from build123d import *

# Parameters (mm, degrees)
F0_R     = 4.5
F0_R_2   = 3
F1_DEPTH = 1.9
F0_R_3   = 6.5
F0_R_4   = 2
F2_DEPTH = 2
F3_R     = 1.75
F5_SIZE  = 0.09999


# Not quite as in the source:
# - a fillet or chamfer is up to 0.001 mm smaller than in the source, because OpenCascade refuses the exact size


with BuildPart() as f1:
    # F0 (on Front) → F1 (new body, symmetric)
    with BuildSketch(Plane.XZ):
        Circle(F0_R)
        Circle(F0_R_2, mode=Mode.SUBTRACT)
    extrude(amount=F1_DEPTH, both=True)

    # F0 (on Front) → F2 (join, symmetric)
    with BuildSketch(Plane.XZ):
        Circle(F0_R_3)
        Circle(F0_R, mode=Mode.SUBTRACT)
        Circle(F0_R_2)
        Circle(F0_R_4, mode=Mode.SUBTRACT)
    extrude(amount=F2_DEPTH, both=True)

    # F4: sweep along a path in F4_path
    with BuildLine(Plane(origin=(6.5, -2, 0), x_dir=(0, 0, -1), z_dir=(0, 1, 0))) as f4_path:
        CenterArc((0, 6.5), 6.5, 0, 360)
    # F3 (on Right) → F4 (sweep, cut)
    with BuildSketch(Plane.YZ):
        with Locations((0, 7.25)):
            Circle(F3_R)
    sweep(path=f4_path.line, mode=Mode.SUBTRACT)

    # F5 (size 0.1 in the source; OpenCascade refuses exactly that, so slightly less here)
    f5_edges = [f1.edges().sort_by_distance(p)[0] for p in [
        (-6.5, -2, 0),
        (-4.5, -2, 0),
        (-3, -1.9, 0),
        (-2, -2, 0),
        (-2, 2, 0),
        (-3, 2, 0),
        (-4.5, 2, 0),
        (-6.5, 2, 0),
    ]]
    chamfer(f5_edges, length=F5_SIZE)


solid = f1.part
Can you work these out from the model? Positions are in its coordinate system, mm. A direction names the side the tool comes from. Give positions to 0.01 mm unless a question says otherwise; leave off trailing zeros. Write each loop counter-clockwise with the first axis right and the second up, starting at its lowest first coordinate (ties: lowest second). Pieces come first, ordered by that corner, then holes. Notation, with made-up numbers: (30, 29) -> (61, 29) arc R18 ccw to (61, 38) -> close; hole circle Ø6 at (-40, 30). An arc over 180 degrees is marked (long way). Answer as a JSON object with one key per item and string values. Group by question number.
Item 1: Suppose I cut it at B-B (y = 0.9). Please give me the cut outline in (x, z), plus the area to 3 significant figures.
Item 2: I'm going to push flat-ended pins straight in: P1, Ø1.5, axis at y = 1, z = 4, coming from the +X side; P2, Ø2.5, axis at x = 0, z = 0, coming from the -Y side. Where does each tip first touch, or does it pass through?
Item 3: Suppose I cut it at A-A (y = 0.15). Please give me the cut outline in (x, z), plus the area to 3 significant figures.
Item 4: Please list where these lines run through material, in increasing order: line 1 (Z direction, x = 0, y = -1.85); line 2 (Y direction, x = 4.25, z = -4.75); line 3 (Z direction, x = 0.25, y = 1.5). Write a range as [from, to].
Item 5: We'd pull the mould along Z, two halves only. Please class faces 3 (the face through (-3.1, -1.9, 1.1)), 4 (the face through (-5.158, -1.743, -3.955)), 5 (the face through (1.3, -2, -2)): +Z half, -Z half, draft (parallel to the pull), parting line (faces both ways), or undercut.
Item 6: For faces 1 (the face through (3, -2, -4)), 2 (the face through (1, 1.9, -3)), which set-ups out of +Z, -Z, +X, -X, +Y, -Y let a thin tool reach every point of the face, with its end or its side?
Findings:
{
 "1": {"outline": "circle Ø11.5 at (0, 0); hole circle Ø4 at (0, 0)", "area": "91.3 mm²"},
 "2": {"P1": "stops at x = 5.46", "P2": "passes through"},
 "3": {"outline": "circle Ø11.01 at (0, 0); hole circle Ø4 at (0, 0)", "area": "82.7 mm²"},
 "4": {"line 1": "z = [-6.5, -2], [2, 6.5]", "line 2": "y = [-2, -1.51], [1.51, 2]", "line 3": "z = [-6.34, -1.98], [1.98, 6.34]"},
 "5": {"face 3": "undercut", "face 4": "parting line", "face 5": "draft"},
 "6": {"face 1": "+Z, -Z, +X, -X, -Y", "face 2": "+Y"}
}
